The listing builds one solid part. Answer for the finished solid, in the listing's coordinates (mm). A direction names the side the tool comes from. Round coordinates to 2 decimals unless told otherwise and drop trailing zeros. Write each loop counter-clockwise with the first axis right and the second up, starting at its lowest first coordinate (ties: lowest second). Pieces come first, ordered by that corner, then holes. Notation, with made-up numbers: (64, -31.75) - (122, -31.75) arc R20 cw to (122, -18.75) - close; hole circle Ø2 at (-2, 63.25). An arc over 180 degrees is marked (long way). Return JSON: item names as keys, results as strings. Group by question number.
(1) Each of these flat-tipped pins is pushed along its axis until it touches: pin 1 (1.5 mm diameter, centred on y = 1.5, z = -13.5, fed in from +X); pin 2 (3 mm diameter, centred on x = -3, z = 3, fed in from -Y); pin 3 (12 mm diameter, centred on x = 1.5, z = -14, fed in from -Y); pin 4 (8 mm diameter, centred on x = 0, y = 0, fed in from -Z). Where does it stop, or does it pass through?
(2) Determine the mould class of faces 1 (the cylindrical face through (0, -3, -7)), 2 (the flat face through (-3.423, 6.024, -10.21)), 3 (the flat face through (2.4, 2.1, 12)), 4 (the cylindrical face through (0.007, 7.845, -9.79)) for opening direction X: +X half, -X half, draft (parallel to the pull), parting line (faces both ways), or undercut.
(3) Section A-A, the plane y = 0 is taken. Write down the section's boundary in (x, z), then the cut area to 3 significant figures.
(4) Section D-D, the plane y = 5.5 is taken. Write down the section's boundary in (x, z), then the cut area to 3 significant figures.
(5) Which of the six approach directions +Z, -Z, +X, -X, +Y, -Y give full straight-line access (tool end or side, diameter ignored) to faces 5 (the flat face through (6.928, 0, -10)), 6 (the cylindrical face through (6.79, 3.93, -9.79)), 7 (the cylindrical face through (6.798, -3.916, -9.79)), 8 (the cylindrical face through (-6.79, -3.93, -9.79)), 9 (the cylindrical face through (0.007, -7.845, -9.79))?
(6) Section B-B, the plane x = 0 is taken. Write down the section's boundary in (y, z), then the cut area to 3 significant figures.
(7) Find the intervals of material crossed by line 1 along X through (y, z) = (0, -11.5); line 2 along Z through (x, y) = (-2.5, -9); line 3 along X through (y, z) = (1, -22.5), in increasing order. Write a range as [from, to].
(8) Section C-C, the plane z = -8 is taken. Write down the section's boundary in (x, y).
```python
from build123d import *

# Parameters (mm, degrees)
CUT_EXTRUDE1_DEPTH = 30
FILLET1_R          = 1


with BuildPart() as part:
    # Sketch2 → Revolve1 (revolve)
    with BuildSketch(Plane(origin=(0, 0, 0), x_dir=(0, 0, -1), z_dir=(1, 0, 0))):
        Polygon((-12, 3), (25, 3), (25, 8), (-5, 8), (-5, 10), (-12, 10), align=None)
    revolve(axis=Axis((0, 0, 0), (0, 0, -1)))

    # Sketch3 → Cut-Extrude1 (cut)
    with BuildSketch(Plane(origin=(0, 0, -25), x_dir=(-1, 0, 0), z_dir=(0, 0, -1))):
        with BuildLine():
            ThreePointArc((0, 8), (-4, 6.92820323), (-6.92820323, 4))
            Line((-6.92820323, 4), (0, 8))
        make_face()
        with BuildLine():
            ThreePointArc((-6.92820323, 4), (-8, 0), (-6.92820323, -4))
            Line((-6.92820323, -4), (-6.92820323, 4))
        make_face()
        with BuildLine():
            ThreePointArc((-6.92820323, -4), (-4, -6.92820323), (0, -8))
            Line((0, -8), (-6.92820323, -4))
        make_face()
        with BuildLine():
            Line((6.92820323, -4), (0, -8))
            ThreePointArc((0, -8), (4, -6.92820323), (6.92820323, -4))
        make_face()
        with BuildLine():
            Line((6.92820323, 4), (6.92820323, -4))
            ThreePointArc((6.92820323, -4), (7.72740661, -2.070552361), (8, 0))
            ThreePointArc((8, 0), (7.72740661, 2.070552361), (6.92820323, 4))
        make_face()
        with BuildLine():
            Line((0, 8), (6.92820323, 4))
            ThreePointArc((6.92820323, 4), (4, 6.92820323), (0, 8))
        make_face()
    extrude(amount=-CUT_EXTRUDE1_DEPTH, mode=Mode.SUBTRACT)

    # Fillet1
    fillet1_edges = [part.edges().sort_by_distance(p)[0] for p in [
        (0, 8, -10),
        (6.92820323, 4, -10),
        (6.92820323, -4, -10),
        (0, -8, -10),
        (-6.92820323, -4, -10),
        (-6.92820323, 4, -10),
    ]]
    fillet(fillet1_edges, radius=FILLET1_R)


solid = part.part
```
Working result:
{
 "1": {"pin 1": "stops at x = 6.93", "pin 2": "stops at y = -7.13", "pin 3": "stops at y = -7.85", "pin 4": "stops at z = -25"},
 "2": {"face 1": "undercut", "face 2": "-X half", "face 3": "draft", "face 4": "parting line"},
 "3": {"outline": "(-10, 5) - (-6.93, 5) - (-6.93, -25) - (-3, -25) - (-3, 12) - (-10, 12) - close; (3, -25) - (6.93, -25) - (6.93, 5) - (10, 5) - (10, 12) - (3, 12) - close", "area": "334 mm^2"},
 "4": {"outline": "(-8.35, 5) - (-4.33, 5) - (-4.33, -25) - (4.33, -25) - (4.33, 5) - (8.35, 5) - (8.35, 12) - (-8.35, 12) - close", "area": "377 mm^2"},
 "5": {"face 5": "-Z, +X, +Y, -Y", "face 6": "-Z, +X, +Y", "face 7": "-Z, +X, -Y", "face 8": "-Z, -X, -Y", "face 9": "-Z, -Y"},
 "6": {"outline": "(-10, 5) - (-7.85, 5) - (-7.85, -25) - (-3, -25) - (-3, 12) - (-10, 12) - close; (3, -25) - (7.85, -25) - (7.85, 5) - (10, 5) - (10, 12) - (3, 12) - close", "area": "389 mm^2"},
 "7": {"line 1": "x = [-6.93, -3], [3, 6.93]", "line 2": "z = [5, 12]", "line 3": "x = [-6.93, -2.83], [2.83, 6.93]"},
 "8": {"outline": "(-6.93, -3.42) arc R1 ccw to (-6.43, -4.29) - (-0.5, -7.71) arc R1 ccw to (0.5, -7.71) - (6.43, -4.29) arc R1 ccw to (6.93, -3.42) - (6.93, 3.42) arc R1 ccw to (6.43, 4.29) - (0.5, 7.71) arc R1 ccw to (-0.5, 7.71) - (-6.43, 4.29) arc R1 ccw to (-6.93, 3.42) - close; hole circle Ø6 at (0, 0)"}
}
